Geometry check sheet. Reference: the model listing, model coordinates, mm. A direction names the side the tool comes from. Give positions to 0.01 mm unless a question says otherwise; leave off trailing zeros. Order: outer loops, then holes, each group sorted by start corner. A loop starts at its lowest first (then second) coordinate and runs counter-clockwise, first axis right, second up. Notation, with made-up numbers: M -25,-27 L 0,-27 A25 ccw 0,6 Z; hole C -4,-18.75 d9. An arc over 180 degrees is marked long. Answer as CSV lines item,"result". Start each with the question number.
Q1. Section check C-C, the plane y = -2. Record the boundary of the cut face in (x, z).
Q2. Section check D-D, the plane z = 84. Record the boundary of the cut face in (x, y).
Q3. Section check B-B, the plane y = -7.75. Record the boundary of the cut face in (x, z).
Q4. Set-up check for faces 5 (the flat face through (-7.952, -1.121, 59.16)), 6 (the flat face through (1.9, -1, 59)), 7 (the cylindrical face through (-1.045, -7.812, 88.513)), 8 (the flat face through (-9.85, -7, 59)), 9 (the flat face through (1, -6.086, 50)): record each of +Z, -Z, +X, -X, +Y, -Y from which the full face is reachable in a straight line by a thin tool's end or side.
Q5. Thickness scan on line 1 (X direction, y = -4.2, z = 10); line 2 (X direction, y = -8.75, z = 70); line 3 (Y direction, x = 1.25, z = 91). Record the ranges inside material, lowest first.
Q6. Section check A-A, the plane z = 50. Record the boundary of the cut face in (x, y), then the cut area to 3 significant figures.
Q7. Go/stop test with flat-tipped pins: pin 1 (1.5 mm diameter, centred on y = -0.5, z = 73, fed in from -X); pin 2 (4.5 mm diameter, centred on x = -0.85, z = 110, fed in from +Y); pin 3 (5 mm diameter, centred on y = 0, z = 23, fed in from +X). Record where each tip stops, or that it passes through.
Q8. Mould release check, pull along Z, two halves, no side actions. Record for faces 1 (the flat face through (1, -6.086, 90)), 2 (the flat face through (-3.6, -1, 59)), 3 (the flat face through (-1, -5, 0)), 4 (the flat face through (-1, -5, 120)): +Z half, -Z half, draft (parallel to the pull), parting line (faces both ways), or undercut.
```python
from build123d import *

# Parameters (mm, degrees)
BOSS_EXTRUDE1_DEPTH = 120
SKETCH2_R           = 2.5
CUT_EXTRUDE1_DEPTH  = 2.5
SKETCH3_R           = 1.5
CUT_EXTRUDE2_DEPTH  = 4.5


with BuildPart() as part:
    # Sketch1 → Boss-Extrude1 (new body)
    with BuildSketch(Plane.XY):
        Polygon((-9.600162866, 1.413680782), (-3.600162866, 1.413680782), (-3.600162866, -3.586319218), (1.899837134, -3.586319218), (1.899837134, 1.413680782), (7.899837134, 1.413680782), (4.649837134, -3.586319218), (8.149837134, -3.586319218), (8.149837134, -9.586319218), (-9.850162866, -9.586319218), (-9.850162866, -3.586319218), (-6.350162866, -3.586319218), align=None)
    extrude(amount=BOSS_EXTRUDE1_DEPTH)

    # Sketch2 → Cut-Extrude1 (cut)
    with BuildSketch(Plane(origin=(0, -3.586319218, 0), x_dir=(1, 0, 0), z_dir=(0, 1, 0))):
        with Locations((-0.850162866, -10)):
            Circle(SKETCH2_R)
        with Locations((-0.850162866, -30)):
            Circle(SKETCH2_R)
        with Locations((-0.850162866, -50)):
            Circle(SKETCH2_R)
        with Locations((-0.850162866, -70)):
            Circle(SKETCH2_R)
        with Locations((-0.850162866, -90)):
            Circle(SKETCH2_R)
        with Locations((-0.850162866, -110)):
            Circle(SKETCH2_R)
    extrude(amount=-CUT_EXTRUDE1_DEPTH, mode=Mode.SUBTRACT)

    # Sketch3 → Cut-Extrude2 (cut, through all)
    with BuildSketch(Plane(origin=(0, -6.086319218, 0), x_dir=(1, 0, 0), z_dir=(0, 1, 0))):
        with Locations((-0.850162866, -10)):
            Circle(SKETCH3_R)
        with Locations((-0.850162866, -30)):
            Circle(SKETCH3_R)
        with Locations((-0.850162866, -50)):
            Circle(SKETCH3_R)
        with Locations((-0.850162866, -70)):
            Circle(SKETCH3_R)
        with Locations((-0.850162866, -90)):
            Circle(SKETCH3_R)
        with Locations((-0.850162866, -110)):
            Circle(SKETCH3_R)
    extrude(amount=-CUT_EXTRUDE2_DEPTH, mode=Mode.SUBTRACT)


solid = part.part
```
Answer block:
1,outline,"M -7.38,0 L -3.6,0 L -3.6,120 L -7.38,120 Z; M 1.9,0 L 5.68,0 L 5.68,120 L 1.9,120 Z"
2,outline,"M -9.85,-9.59 L 8.15,-9.59 L 8.15,-3.59 L 4.65,-3.59 L 7.9,1.41 L 1.9,1.41 L 1.9,-3.59 L -3.6,-3.59 L -3.6,1.41 L -9.6,1.41 L -6.35,-3.59 L -9.85,-3.59 Z"
3,outline,"M -9.85,0 L 8.15,0 L 8.15,120 L -9.85,120 Z; hole C -0.85,10 d3; hole C -0.85,30 d3; hole C -0.85,50 d3; hole C -0.85,70 d3; hole C -0.85,90 d3; hole C -0.85,110 d3"
4,face 5,"+Z, -Z, -X"
4,face 6,"+Z, -Z, +Y"
4,face 7,"+Y, -Y"
4,face 8,"+Z, -Z, -X, +Y, -Y"
4,face 9,"+Y"
5,line 1,"x = -9.85 to -3.35, 1.65 to 8.15"
5,line 2,"x = -9.85 to -2.35, 0.65 to 8.15"
5,line 3,"y = -9.59 to -6.09"
6,outline,"M -9.85,-9.59 L -2.35,-9.59 L -2.35,-6.09 L -3.35,-6.09 L -3.35,-3.59 L -3.6,-3.59 L -3.6,1.41 L -9.6,1.41 L -6.35,-3.59 L -9.85,-3.59 Z; M 0.65,-9.59 L 8.15,-9.59 L 8.15,-3.59 L 4.65,-3.59 L 7.9,1.41 L 1.9,1.41 L 1.9,-3.59 L 1.65,-3.59 L 1.65,-6.09 L 0.65,-6.09 Z"
6,area,"129 mm2"
7,pin 1,"stops at x = -8.84"
7,pin 2,"stops at y = -6.09"
7,pin 3,"stops at x = 7.9"
8,face 1,"undercut"
8,face 2,"draft"
8,face 3,"-Z half"
8,face 4,"+Z half"
